Part model, mm, in its own coordinate system. Face numbers are marked on the shaded views. A direction names the side the tool comes from. Give positions to 0.01 mm unless a question says otherwise; leave off trailing zeros. Loops run counter-clockwise (first coordinate to the right, second up) from the corner with the lowest first, then second, coordinate; pieces in that order, holes last. Notation, with made-up numbers: (-7.5, 77.25) -> (1.5, 77.25) arc R29 ccw to (1.5, 111.25) -> close; hole circle Ø9 at (-8, 39.5). An arc over 180 degrees is marked (long way). Write item = value, one per line.
from build123d import *

# Parameters (mm, degrees)
BOSS_EXTRUDE2_DEPTH = 6.35
SKETCH4_R           = 3.81
CUT_EXTRUDE1_DEPTH  = 12.7
CUT_EXTRUDE2_DEPTH  = 3.81


with BuildPart() as part:
    # Sketch3 → Boss-Extrude2 (new body)
    with BuildSketch(Plane(origin=(0, 0, 0), x_dir=(1, 0, 0), z_dir=(0, 1, 0))):
        with BuildLine():
            Line((-15.875, 7.62), (15.875, 7.62))
            ThreePointArc((15.875, 7.62), (17.609089272, 0), (15.875, -7.62))
            Line((15.875, -7.62), (-15.875, -7.62))
            ThreePointArc((-15.875, -7.62), (-17.609089272, 0), (-15.875, 7.62))
        make_face()
    extrude(amount=BOSS_EXTRUDE2_DEPTH)

    # Sketch4 → Cut-Extrude1 (cut)
    with BuildSketch(Plane(origin=(0, 6.35, 0), x_dir=(1, 0, 0), z_dir=(0, 1, 0))):
        with Locations((12.065, 0)):
            Circle(SKETCH4_R)
        with Locations((-12.065, 0)):
            Circle(SKETCH4_R)
    extrude(amount=-CUT_EXTRUDE1_DEPTH, mode=Mode.SUBTRACT)

    # Sketch5 → Cut-Extrude2 (cut)
    with BuildSketch(Plane.XZ):
        with BuildLine():
            Line((15.875, 7.62), (-0.635, 7.62))
            Line((-0.635, 7.62), (-0.635, -7.62))
            Line((-0.635, -7.62), (15.875, -7.62))
            ThreePointArc((15.875, -7.62), (17.609089272, 0), (15.875, 7.62))
        make_face()
    extrude(amount=-CUT_EXTRUDE2_DEPTH, mode=Mode.SUBTRACT)


solid = part.part
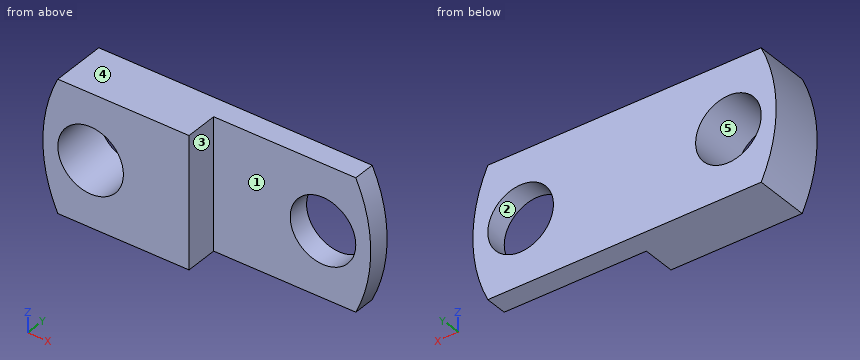
1) Drill centre lines: line 1 along Y through (x, z) = (4, -2.5); line 2 along X through (y, z) = (3, 2.25) (3 decimals); line 3 along Z through (x, y) = (-10.5, 4.5). Where is each one in solid material? Low to high. Write a range as [from, to].
Resolved:
line_1 = [3.81, 6.35]
line_2 = [-17.465, -15.14], [-8.99, -0.635]
line_3 = [-7.62, -3.47], [3.47, 7.62]
2) Slice it at C-C, the plane x = 14. List the corners of the cut face in (y, z), and give its area (3 significant figures).
Resolved:
outline = (3.81, -7.62) -> (6.35, -7.62) -> (6.35, -3.28) -> (3.81, -3.28) -> close; (3.81, 3.28) -> (6.35, 3.28) -> (6.35, 7.62) -> (3.81, 7.62) -> close
area = 22.0 mm²
3) Pull direction X, two halves, no side cores. Call the marked faces 3, 4 and 5: pulls with the +X half, pulls with the -X half, needs draft (parallel to the pull), parting line crosses it, or undercut.
Resolved:
face_3 = pulls with the +X half
face_4 = needs draft
face_5 = undercut
4) Slice it at B-B, the plane z = 0. List the corners of the cut face in (x, y) (3 decimals).
Resolved:
outline = (-17.609, 0) -> (-15.875, 0) -> (-15.875, 6.35) -> (-17.609, 6.35) -> close; (-8.255, 0) -> (-0.635, 0) -> (-0.635, 3.81) -> (8.255, 3.81) -> (8.255, 6.35) -> (-8.255, 6.35) -> close; (15.875, 3.81) -> (17.609, 3.81) -> (17.609, 6.35) -> (15.875, 6.35) -> close
5) Slice it at A-A, the plane y = 4.5. List the corners of the cut face in (x, z) (3 decimals).
Resolved:
outline = (-15.875, -7.62) -> (15.875, -7.62) arc R17.609 ccw to (15.875, 7.62) -> (-15.875, 7.62) arc R17.609 ccw to start; hole circle Ø7.62 at (-12.065, 0); hole circle Ø7.62 at (12.065, 0)
6) Which spindle directions (+Z, -Z, +X, -X, +Y, -Y) get a long thin tool onto all of the face, cutting with end or side? Do the marked faces 1 and 2. Say none if no direction does.
Resolved:
face_1 = +Z, -Z, +X, -Y
face_2 = +Y, -Y
7) Slice it at D-D, the plane y = 2.75. List the corners of the cut face in (x, z) (3 decimals), and give its area (3 significant figures).
Resolved:
outline = (-15.875, -7.62) -> (-0.635, -7.62) -> (-0.635, 7.62) -> (-15.875, 7.62) arc R17.609 ccw to start; hole circle Ø7.62 at (-12.065, 0)
area = 204 mm²
8) Drop flat-ended pins along their axis: P1, Ø4.5, axis at x = 12.065, z = 0, coming from the -Y side; P2, Ø1.5, axis at y = 2.5, z = -5.5, coming from the -X side; P3, Ø4.5, axis at x = 5.5, z = -0.5, coming from the -Y side. Give the stop position or say it passes through.
Resolved:
P1 = through
P2 = -16.96
P3 = 3.81
